Autodesk Fusion 360 part; units mm, degrees
sketch "Sketch1" plane through (0, 0, 0) normal (0, 0, 1) x (1, 0, 0)
  line L0 (0, 0) -> (152.4, 0)
  line L1 (152.4, 0) -> (152.4, 57.15)
  line L2 (152.4, 57.15) -> (0, 57.15)
  line L3 (0, 57.15) -> (0, 0)
  circle A0 centre (6.35, 6.35) radius 1.985
  circle A1 centre (146.05, 6.35) radius 1.985
  circle A2 centre (6.35, 50.8) radius 1.985
  circle A3 centre (146.05, 50.8) radius 1.985
  circle A4 centre (6.35, 6.35) radius 1.985
  circle A5 centre (6.35, 28.575) radius 1.985
  circle A6 centre (146.05, 28.575) radius 1.985
  circle A7 centre (76.2, 6.35) radius 1.985
  circle A8 centre (38.1, 6.35) radius 1.985
  circle A9 centre (114.3, 6.35) radius 1.985
  circle A10 centre (38.1, 50.8) radius 1.985
  circle A11 centre (76.2, 50.8) radius 1.985
  circle A12 centre (114.3, 50.8) radius 1.985
  point P0 (6.35, 6.35)
  dimension "d1" = 57.15
  dimension "d2" = 152.4
  dimension "d3" = 3.97
  dimension "d4" = 3.97
  dimension "d5" = 3.97
  dimension "d6" = 3.97
  dimension "d10" = 3.97
  dimension "d11" = 3.97
  dimension "d12" = 3.97
  dimension "d13" = 3.97
  dimension "d14" = 3.97
  dimension "d15" = 3.97
  dimension "d16" = 3.97
  dimension "d17" = 3.97
  dimension "d18" = 3.97
extrude "Extrude1" add sketch "Sketch1" against normal blind 6.35
Geometry check sheet. Reference: the model listing, model coordinates, mm. Coordinates: 2 decimals unless noted, no trailing zeros. Order: outer loops, then holes, each group sorted by start corner. A loop starts at its lowest first (then second) coordinate and runs counter-clockwise, first axis right, second up. Notation, with made-up numbers: (-18, -14) - (21, -14) arc R17 cw to (21, 18) - close; hole circle Ø3 at (22, 34.25). An arc over 180 degrees is marked (long way). Answer as a JSON object with one key per item and string values. Group by question number.
Item 1: Sectioned sample at B-B, the plane y = 6.35. Record the cut outline in (x, z) (3 decimals), and give its area (3 significant figures).
Item 2: Sectioned sample at C-C, the plane x = 76.2. Record the cut outline in (y, z) (3 decimals).
Item 3: Scan lines: probe 1 along Y at (x, z) = (146.05, -4) (3 decimals); probe 2 along Y at (x, z) = (38.1, -3) (3 decimals); probe 3 along X at (y, z) = (8, -2). Record each from-to range of solid material in increasing order.
Item 4: Draft check along Y on faces 1 (the face through (152.4, 28, -3)), 2 (the face through (75, 0, -3)), 3 (the face through (39.934, 50.04, -3.131)). Enter one of: +Y half, -Y half, draft (parallel to the pull), parting line (faces both ways), or undercut.
Item 5: Sectioned sample at D-D, the plane z = -4.5. Give the number of separate pieces and of enclosed holes in the cut face, and give its area (3 significant figures).
Item 6: Sectioned sample at A-A, the plane x = 6.35. Record the cut outline in (y, z) (3 decimals).
Item 7: Depth check by flat-ended pin: pin 1 Ø3 at (x, y) = (114.3, 6.35) entering from +Z. Enter the tip coordinate at first touch or a pass-through.
Resolved:
{
 "1": {"outline": "(0, -6.35) - (4.365, -6.35) - (4.365, 0) - (0, 0) - close; (8.335, -6.35) - (36.115, -6.35) - (36.115, 0) - (8.335, 0) - close; (40.085, -6.35) - (74.215, -6.35) - (74.215, 0) - (40.085, 0) - close; (78.185, -6.35) - (112.315, -6.35) - (112.315, 0) - (78.185, 0) - close; (116.285, -6.35) - (144.065, -6.35) - (144.065, 0) - (116.285, 0) - close; (148.035, -6.35) - (152.4, -6.35) - (152.4, 0) - (148.035, 0) - close", "area": "842 mm^2"},
 "2": {"outline": "(0, -6.35) - (4.365, -6.35) - (4.365, 0) - (0, 0) - close; (8.335, -6.35) - (48.815, -6.35) - (48.815, 0) - (8.335, 0) - close; (52.785, -6.35) - (57.15, -6.35) - (57.15, 0) - (52.785, 0) - close"},
 "3": {"probe 1": "0 to 4.365, 8.335 to 26.59, 30.56 to 48.815, 52.785 to 57.15", "probe 2": "0 to 4.365, 8.335 to 48.815, 52.785 to 57.15", "probe 3": "0 to 5.25, 7.45 to 37, 39.2 to 75.1, 77.3 to 113.2, 115.4 to 144.95, 147.15 to 152.4"},
 "4": {"face 1": "draft", "face 2": "-Y half", "face 3": "undercut"},
 "5": {"separate pieces": "1", "enclosed holes": "12", "area": "8,560 mm^2"},
 "6": {"outline": "(0, -6.35) - (4.365, -6.35) - (4.365, 0) - (0, 0) - close; (8.335, -6.35) - (26.59, -6.35) - (26.59, 0) - (8.335, 0) - close; (30.56, -6.35) - (48.815, -6.35) - (48.815, 0) - (30.56, 0) - close; (52.785, -6.35) - (57.15, -6.35) - (57.15, 0) - (52.785, 0) - close"},
 "7": {"pin 1": "through"}
}
